The figure shows three views and two pictorial views of one solid part (mm, origin at its lowest corner). Answer the questions. Round coordinates to 2 decimals unless told otherwise and drop trailing zeros. Order: outer loops, then holes, each group sorted by start corner. A loop starts at its lowest first (then second) coordinate and runs counter-clockwise, first axis right, second up. Notation, with made-up numbers: (-28, -17.5) - (24, -17.5) arc R26 cw to (24, 19.5) - close; hole circle Ø2 at (73.5, 10.5). An arc over 180 degrees is marked (long way). Write item = value, one per line.
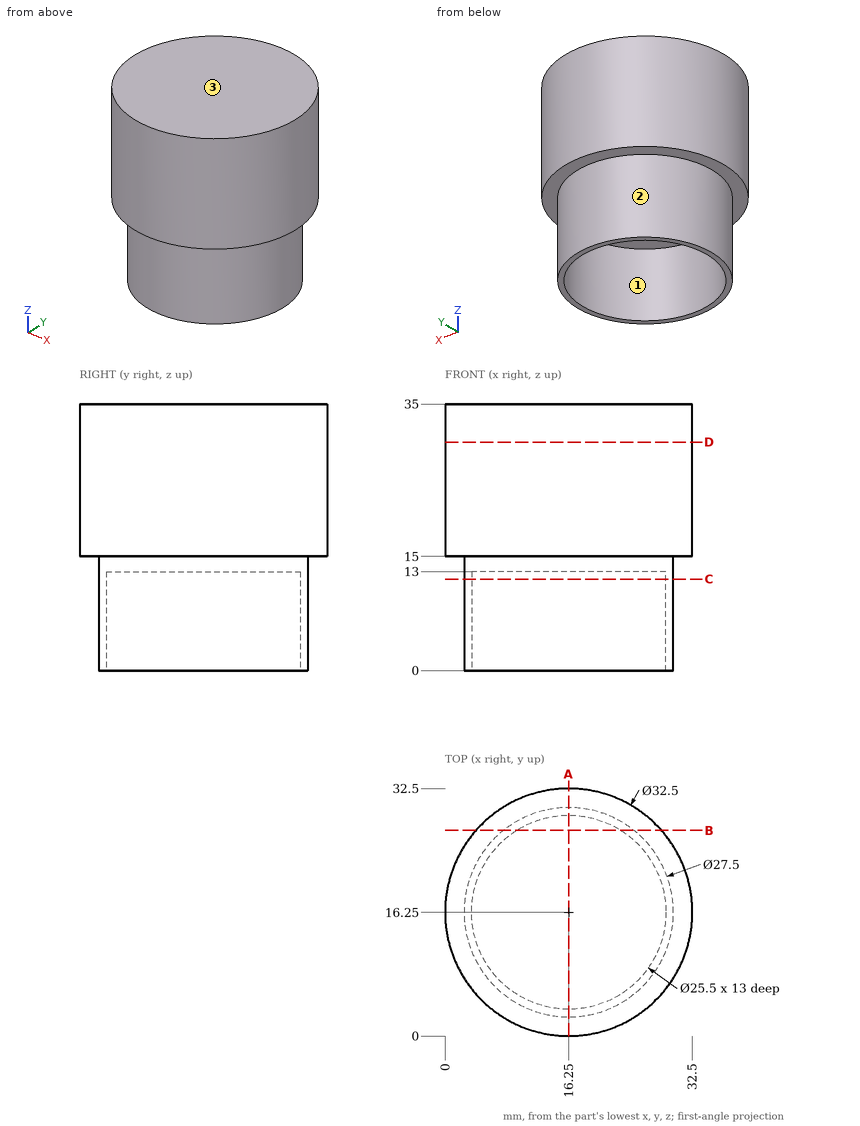
Q1. Flat-ended cylindrical pins translate along their axes: P1, Ø3, axis at x = 17, y = 25, coming from the -Z side; P2, Ø8, axis at x = 26.5, z = 31, coming from the -Y side; P3, Ø4, axis at y = 18.5, z = 25, coming from the +X side; P4, Ø13, axis at x = 12.5, y = 10.5, coming from the -Z side. Find the tip coordinate at first contact, or state that the pin passes through.
Model answer:
P1 = 13
P2 = 1.25
P3 = 32.5
P4 = 0
Q2. Section A-A on x = 16.25 is taken. Determine the outline of the cut face in (y, z).
Model answer:
outline = (0, 15) - (2.5, 15) - (2.5, 0) - (3.5, 0) - (3.5, 13) - (29, 13) - (29, 0) - (30, 0) - (30, 15) - (32.5, 15) - (32.5, 35) - (0, 35) - close
Q3. Section D-D on z = 30 is taken. Determine the outline of the cut face in (x, y).
Model answer:
outline = circle Ø32.5 at (16.25, 16.25)
Q4. Section B-B on y = 27 is taken. Determine the outline of the cut face in (x, z).
Model answer:
outline = (4.06, 15) - (7.68, 15) - (7.68, 0) - (9.39, 0) - (9.39, 13) - (23.11, 13) - (23.11, 0) - (24.82, 0) - (24.82, 15) - (28.44, 15) - (28.44, 35) - (4.06, 35) - close
Q5. Section C-C on z = 12 is taken. Determine the outline of the cut face in (x, y).
Model answer:
outline = circle Ø27.5 at (16.25, 16.25); hole circle Ø25.5 at (16.25, 16.25)
Q6. Determine the mould class of the marked faces 1, 2 and 3 for opening direction X: released by +X, released by -X, zero draft, split by the parting line, or undercut.
Model answer:
face_1 = undercut
face_2 = split by the parting line
face_3 = zero draft
Q7. Find the intervals of material crossed by line 1 (Y direction, x = 16.25, z = 5); line 2 (Z direction, x = 30, y = 18), in increasing order. Write a range as from..to.
Model answer:
line_1 = 2.5..3.5, 29..30
line_2 = 15..35
